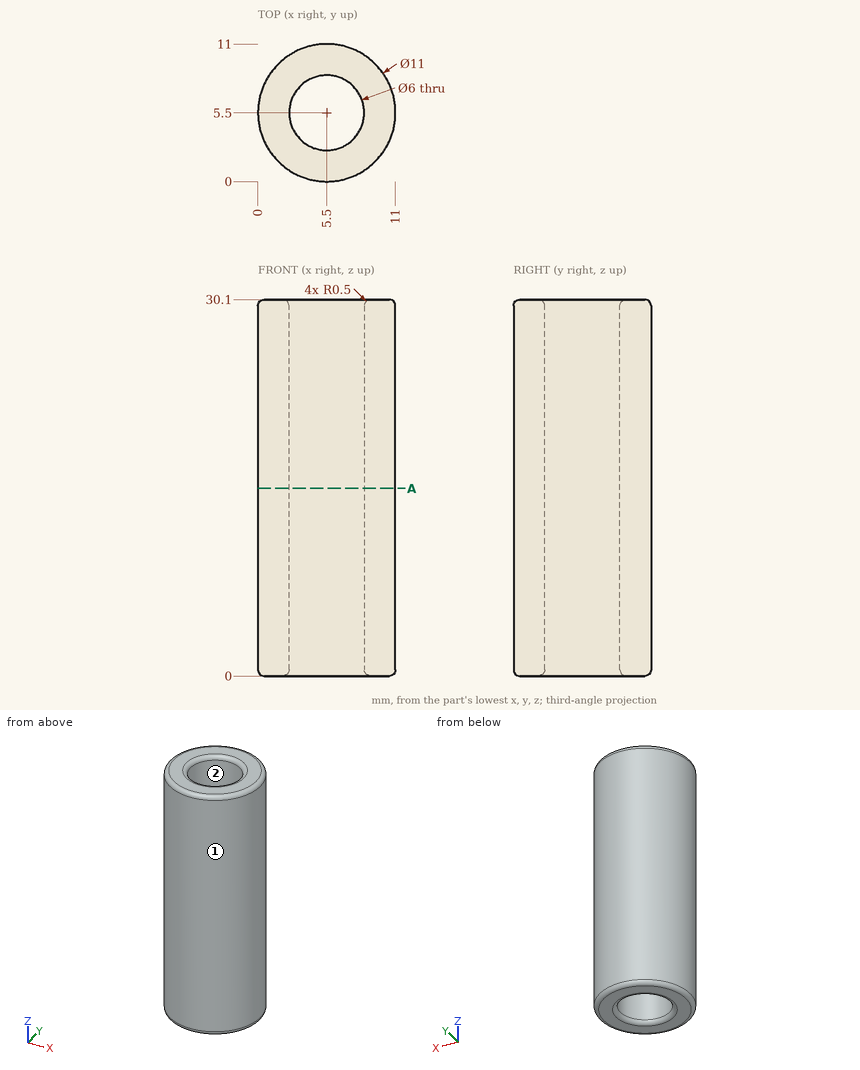
Print and shaded views of the part. All mm, measured from the part's lowest x, y and z. Coordinates: 2 decimals unless noted, no trailing zeros. Order: outer loops, then holes, each group sorted by start corner. A loop starts at its lowest first (then second) coordinate and runs counter-clockwise, first axis right, second up.
(1) Probe L1, parallel to Y at x = 5.5, z = 19; L2, parallel to X at y = 4, z = 16.5; L3, parallel to X at y = 8.25, z = 2. List the from-to ranges inside material, lowest first.
Check sheet entries:
L1: y = 0 to 2.5, 8.5 to 11
L2: x = 0.21 to 2.9, 8.1 to 10.79
L3: x = 0.74 to 4.3, 6.7 to 10.26
(2) Pin check, flat tips, straight feed: pin 1 Ø1.5 at (x, y) = (5, 7) entering from -Z; pin 2 Ø2 at (y, z) = (6, 9.5) entering from -X; pin 3 Ø2 at (x, z) = (7.5, 17) entering from -Y; pin 4 Ø1 at (y, z) = (2, 20) entering from -X. Stop position of each tip, or through.
Check sheet entries:
pin 1: passes through
pin 2: stops at x = 0
pin 3: stops at y = 0.09
pin 4: stops at x = 0.89
(3) Pull direction X, two halves, no side cores. Call the marked faces 1 and 2: pulls with the +X half, pulls with the -X half, needs draft (parallel to the pull), parting line crosses it, or undercut.
Check sheet entries:
face 1: parting line crosses it
face 2: undercut
(4) Slice it at A-A, the plane z = 15. Write the cut outline in (x, y), and give its area (3 significant figures).
Check sheet entries:
outline: circle Ø11 at (5.5, 5.5); hole circle Ø6 at (5.5, 5.5)
area: 66.8 mm2
